The listing builds one solid part. Answer for the finished solid, in the listing's coordinates (mm). Face numbers are marked on the shaded views. A direction names the side the tool comes from. Coordinates: 2 decimals unless noted, no trailing zeros. Write each loop counter-clockwise with the first axis right and the second up, starting at its lowest first coordinate (ties: lowest second). Pieces come first, ordered by that corner, then holes. Notation, with made-up numbers: M 4,33 L 17,33 A17 cw 17,54 Z; hole C 80,-21 d6. An arc over 180 degrees is marked long. Answer as CSV lines item,"result".
```python
from build123d import *

# Parameters (mm, degrees)
F0_R     = 12
F1_DEPTH = 26
F2_R     = 12
F3_DEPTH = 9
F5_DEPTH = 15
F7_W     = 12
F7_H     = 17
F8_DEPTH = 6.425


with BuildPart() as f1:
    # F0 (on Top) → F1 (new body)
    with BuildSketch(Plane.XY):
        Circle(F0_R)
    extrude(amount=F1_DEPTH)

    # F2 (on face) → F3 (cut)
    with BuildSketch(Plane.XY.offset(26)):
        Circle(F2_R)
        with BuildLine():
            ThreePointArc((-3.462659053, -2.6329626437), (-1.3892323635, 4.1222000728), (4.35, 0))
            ThreePointArc((4.35, 0), (4.1222000728, -1.3892323635), (3.462659053, -2.6329626437))
            ThreePointArc((3.462659053, -2.6329626437), (0, -8.215), (-3.462659053, -2.6329626437))
        make_face(mode=Mode.SUBTRACT)
        with BuildLine():
            ThreePointArc((3.462659053, -2.6329626437), (4.1222000728, -1.3892323635), (4.35, 0))
            ThreePointArc((4.35, 0), (-1.3892323635, 4.1222000728), (-3.462659053, -2.6329626437))
            ThreePointArc((-3.462659053, -2.6329626437), (0, -4.35), (3.462659053, -2.6329626437))
        make_face()
    extrude(amount=-F3_DEPTH, mode=Mode.SUBTRACT)

    # F4 (on face) → F5 (cut)
    with BuildSketch(Plane.XY.offset(17)):
        with BuildLine():
            ThreePointArc((3.462659053, -2.6329626437), (4.1222000728, -1.3892323635), (4.35, 0))
            ThreePointArc((4.35, 0), (-1.3892323635, 4.1222000728), (-3.462659053, -2.6329626437))
            ThreePointArc((-3.462659053, -2.6329626437), (0, -4.35), (3.462659053, -2.6329626437))
        make_face()
    extrude(amount=-F5_DEPTH, mode=Mode.SUBTRACT)

    # F7 (on offset) → F8 (cut)
    with BuildSketch(Plane.XZ.offset(-12)):
        with Locations((6, 8.5)):
            Rectangle(F7_W, F7_H)
        with Locations((-6, 8.5)):
            Rectangle(F7_W, F7_H)
    extrude(amount=F8_DEPTH, mode=Mode.SUBTRACT)


solid = f1.part
```
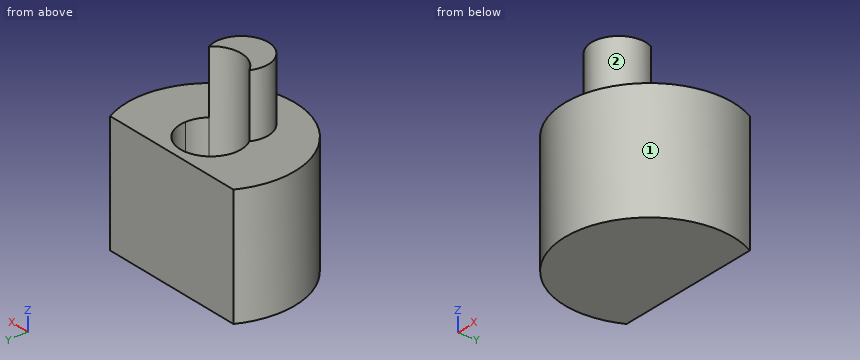
Q1. For the marked faces 1 and 2, determine the directions among +Z, -Z, +X, -X, +Y, -Y from which every point of the face is accessible in a straight line to the end or side of a thin tool.
Output:
face 1,"+Z, -Z"
face 2,"+Z"
Q2. Find section D-D (z = 23.75). Give the vertices of the cut face in (x, y) (3 decimals).
Output:
outline,"M -3.463,-2.633 A3.865 ccw long 3.463,-2.633 A4.35 cw Z"
Q3. Find section B-B (x = 0). Give the vertices of the cut face in (y, z) (3 decimals), and give its area (3 significant figures).
Output:
outline,"M -12,0 L 5.575,0 L 5.575,17 L 4.35,17 L 4.35,2 L -4.35,2 L -4.35,26 L -8.215,26 L -8.215,17 L -12,17 Z"
area,"203 mm2"
Q4. Find section A-A (z = 8.5). Give the vertices of the cut face in (x, y) (3 decimals).
Output:
outline,"M -10.626,5.575 A12 ccw long 10.626,5.575 Z; hole C 0,0 d8.7"
Q5. Flat-ended cylindrical pins translate along their axes: pin 1 Ø2 at (y, z) = (-7.5, 4.5) entering from -X; pin 2 Ø4 at (x, y) = (-4.5, -8.5) entering from +Z; pin 3 Ø10 at (x, z) = (-5, 22.5) entering from +Y. Find the tip coordinate at first contact, or state that the pin passes through.
Output:
pin 1,"x = -10.09"
pin 2,"z = 17"
pin 3,"y = -2.63"
Q6. Find section C-C (y = -2). Give the vertices of the cut face in (x, z), and give its area (3 significant figures).
Output:
outline,"M -11.83,0 L 11.83,0 L 11.83,17 L 3.86,17 L 3.86,2 L -3.86,2 L -3.86,17 L -11.83,17 Z"
area,"286 mm2"
Q7. Straight lines are drawn through the part: line 1 (Z direction, x = -5.25, y = -3); line 2 (Y direction, x = -3.25, z = 15) (3 decimals); line 3 (X direction, y = 1.75, z = 14.25). For each, find the intervals that lie inside material, in ascending order.
Output:
line 1,"0 to 17"
line 2,"-11.552 to -2.891, 2.891 to 5.575"
line 3,"-11.87 to -3.98, 3.98 to 11.87"
